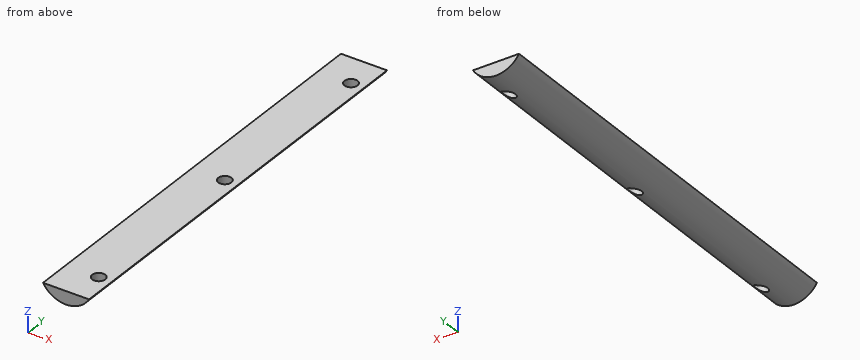
```python
from build123d import *

# Parameters (mm, degrees)
BOSS_EXTRUDE1_START     = -6.35
BOSS_EXTRUDE1_DEPTH     = 209.972402
SKETCH1_R               = 3.175
CUT_EXTRUDE2_DEPTH      = 1
CUT_EXTRUDE2_DEPTH_BACK = 7.35


with BuildPart() as part:
    # Sketch2 → Boss-Extrude1 (new body)
    with BuildSketch(Plane(origin=(0, 0, 0), x_dir=(1, 0, 0), z_dir=(0, 1, 0)).offset(BOSS_EXTRUDE1_START)):
        with BuildLine():
            Line((0, 0), (6.35, 0))
            ThreePointArc((6.35, 0), (-4.7625, 6.35), (-15.875, 0))
            Line((-15.875, 0), (0, 0))
        make_face()
    extrude(amount=BOSS_EXTRUDE1_DEPTH)

    # Sketch1 → Cut-Extrude2 (cut, two sides)
    with BuildSketch(Plane.XY) as cut_extrude2_sk:
        with Locations((0, 187.536328)):
            Circle(SKETCH1_R)
        with Locations((0, 9.736074)):
            Circle(SKETCH1_R)
        with Locations((0, 98.636201)):
            Circle(SKETCH1_R)
    extrude(amount=CUT_EXTRUDE2_DEPTH, mode=Mode.SUBTRACT)
    extrude(cut_extrude2_sk.sketch, amount=-CUT_EXTRUDE2_DEPTH_BACK, mode=Mode.SUBTRACT)


solid = part.part
```
For this review, take the finished solid that the model builds, in its own axes (mm). Give positions to 0.01 mm unless a question says otherwise; leave off trailing zeros. Write each loop counter-clockwise with the first axis right and the second up, starting at its lowest first coordinate (ties: lowest second). Pieces come first, ordered by that corner, then holes. Notation, with made-up numbers: M -15,28 L 26,28 A22 cw 26,48 Z; hole C 35.5,-4.75 d3. An arc over 180 degrees is marked long. Answer as a JSON object with one key per item and string values. Group by question number.
Item 1: Consider section A-A on z = -1.25. Write out the cut boundary in (x, y) (3 decimals), plus the area to 3 significant figures.
Item 2: Consider section D-D on x = -11.75. Write out the cut boundary in (y, z).
Item 3: For probe 1 along Y at (x, z) = (0, -2.5); probe 2 along Y at (x, z) = (-2, -3.25); probe 3 along X at (y, z) = (8.5, -3), list the stretches that pass through material, from the lowest coordinate up. Write a range as [from, to].
Item 4: For pin 1 Ø1 at (y, z) = (15.5, -2.5) entering from +X; pin 2 Ø7.5 at (x, y) = (0, 9.74) entering from -Z; pin 3 Ø4 at (x, y) = (0, 98.64) entering from +Z; pin 4 Ø2 at (y, z) = (101, -4) entering from -X, all flat-tipped, find the tip position at first contact; note any pin that passes through.
Item 5: Consider section B-B on x = 0. Write out the cut boundary in (y, z).
Check result:
{
 "1": {"outline": "M -15.036,-6.35 L 5.511,-6.35 L 5.511,203.622 L -15.036,203.622 Z; hole C 0,9.736 d6.35; hole C 0,98.636 d6.35; hole C 0,187.536 d6.35", "area": "4,220 mm^2"},
 "2": {"outline": "M -6.35,-4.29 L 203.62,-4.29 L 203.62,0 L -6.35,0 Z"},
 "3": {"probe 1": "y = [-6.35, 6.56], [12.91, 95.46], [101.81, 184.36], [190.71, 203.62]", "probe 2": "y = [-6.35, 7.27], [12.2, 96.17], [101.1, 185.07], [190, 203.62]", "probe 3": "x = [-13.43, -2.92], [2.92, 3.91]"},
 "4": {"pin 1": "stops at x = 4.9", "pin 2": "stops at z = -6.31", "pin 3": "passes through", "pin 4": "stops at x = -13.43"},
 "5": {"outline": "M -6.35,-5.44 L 6.56,-5.44 L 6.56,0 L -6.35,0 Z; M 12.91,-5.44 L 95.46,-5.44 L 95.46,0 L 12.91,0 Z; M 101.81,-5.44 L 184.36,-5.44 L 184.36,0 L 101.81,0 Z; M 190.71,-5.44 L 203.62,-5.44 L 203.62,0 L 190.71,0 Z"}
}
